Autodesk Inventor part; units mm, degrees
ref_plane "YZ Plane" through (0, 0, 0) normal (1, 0, 0) x (0, 1, 0)
ref_plane "XZ Plane" through (0, 0, 0) normal (0, 1, 0) x (-1, 0, 0)
ref_plane "XY Plane" through (0, 0, 0) normal (0, 0, 1) x (1, 0, 0)
sketch "Sketch1" plane through (0, 0, 0) normal (0, 0, 1) x (1, 0, 0)
  line L0 (0, 0) -> (25, 0)
  line L1 (25, 0) -> (25, 3)
  line L2 (0, 3) -> (25, 3)
  line L3 (0, 0) -> (0, 3)
  line L4 (0.2071, -72) -> (11, -72)
  line L5 (0.2071, -69) -> (11, -69)
  line L6 (25, -69) -> (50, -69)
  line L7 (25, 0) -> (50, 0)
  line L8 (-25, 0) -> (0, 0)
  line L9 (-22, 0) -> (-22, -10.8146)
  line L10 (-25, -22) -> (-25, -47)
  line L11 (-25, -47) -> (-22, -47)
  line L12 (-22, -10.8146) -> (-22, -58.1854)
  line L13 (-25, -22) -> (-22, -22)
  line L14 (-22, -58.1854) -> (-22, -69)
  line L15 (-25, -69) -> (0, -69)
  line L16 (50, 0) -> (50, -22)
  line L17 (50, -22) -> (47, -22)
  line L18 (47, -22) -> (47, -47)
  line L19 (47, -47) -> (50, -47)
  line L20 (50, -47) -> (50, -69)
  line L21 (50, 0) -> (25, 0)
  line L22 (25, 3) -> (25, 0)
  line L23 (25, 3) -> (0, 3)
  line L24 (0, 3) -> (0, 0)
  line L25 (-22, -10.8146) -> (-22, 0)
  line L26 (-22, 0) -> (0, 0)
  line L27 (-22, -22) -> (-25, -22)
  line L28 (-25, -22) -> (-25, -47)
  line L29 (-22, -47) -> (-25, -47)
  line L30 (-22, -58.1854) -> (-22, -69)
  line L31 (-22, -69) -> (0, -69)
  line L32 (0, -72) -> (0, -69)
  line L33 (0, -72) -> (25, -72)
  line L34 (25, -72) -> (25, -69)
  line L35 (25, -69) -> (50, -69)
  line L36 (11, -72) -> (11, -69)
  line L37 (0.2071, -69) -> (0.2071, -72)
  dimension "d0" = 3
extrude "Extrusion1" add sketch "Sketch1" along normal blind 3
sketch "Sketch2" plane through (0, 0, 3) normal (0, 0, 1) x (1, 0, 0)
  line L0 (-25, -22) -> (-25, -47)
  line L1 (-25, -34.5) -> (7, -34.5)
  line L2 (-25, -34.5) -> (-14, -34.5)
  circle A0 centre (-14, -34.5) radius 21
  circle A1 centre (-14, -34.5) radius 25
  point P0 (0, 0)
  dimension "d3" = 32
  dimension "d4" = 11
  dimension "d5" = 4
extrude "Extrusion2" cut sketch "Sketch2" against normal blind 20 contours A0 | A1
sketch "Sketch3" plane through (0, 0, 3) normal (0, 0, 1) x (1, 0, 0)
  line L0 (-1.2929, -65) -> (30.2929, -65)
  line L1 (-4.5, -67) -> (-4.5, -65)
  line L2 (33.5, -67) -> (33.5, -65)
  line L3 (30.6464, -65) -> (33.5, -65)
  line L4 (30.6464, -65) -> (30.2929, -65)
  line L5 (30.2929, -67) -> (30.6464, -67)
  line L6 (33.5, -67) -> (30.6464, -67)
  line L7 (30.2929, -67) -> (-1.2929, -67)
  arc A0 (-22, -58.1854) -> (-22, -10.8146) centre (-14, -34.5) ccw
  line L8 (-22, -58.1854) -> (-22, -69)
  line L9 (-22, -69) -> (0, -69)
  line L10 (0, -69) -> (0, -72)
  line L11 (50, -69) -> (50, -47)
  line L12 (50, -47) -> (47, -47)
  line L13 (47, -47) -> (47, -22)
  line L14 (47, -22) -> (50, -22)
  line L15 (50, -22) -> (50, 0)
  line L16 (50, 0) -> (25, 0)
  line L17 (25, 0) -> (25, 3)
  line L18 (25, 3) -> (0, 3)
  line L19 (0, 3) -> (0, 0)
  line L20 (0, 0) -> (-22, 0)
  line L21 (-22, 0) -> (-22, -10.8146)
  line L22 (-4.5, -65) -> (-1.6464, -65)
  line L23 (-1.2929, -65) -> (-1.6464, -65)
  line L24 (-1.6464, -67) -> (-4.5, -67)
  line L25 (-1.6464, -67) -> (-1.2929, -67)
  line L26 (0, -72) -> (25, -72)
  line L27 (25, -69) -> (50, -69)
  line L28 (25, -72) -> (25, -69)
extrude "Extrusion3" cut sketch "Sketch3" against normal blind 3 contours L0 L4 L3 L2 L6 L5 L7 L25 L24 L1 L22 L23
sketch "Sketch4" plane through (0, 0, 3) normal (0, 0, 1) x (1, 0, 0)
  line L0 (47, -47) -> (47, -22)
  line L1 (47, -34.5) -> (34.3, -34.5)
  line L2 (34.3, -34.5) -> (34.3, -36)
  line L3 (34.3, -36) -> (34.3, -33)
  line L4 (34.3, -33) -> (47, -33)
  line L5 (47, -33) -> (47, -36)
  line L6 (47, -36) -> (34.3, -36)
  line L7 (40.65, -36) -> (40.65, -38)
  line L8 (40.65, -38) -> (38.15, -38)
  line L9 (38.15, -38) -> (38.15, -31)
  line L10 (38.15, -31) -> (40.65, -31)
  line L11 (40.65, -31) -> (40.65, -36)
  line L12 (25, 3) -> (0, 3)
  line L13 (50, 0) -> (25, 0)
  line L14 (0, 0) -> (-22, 0)
  line L15 (25, -69) -> (50, -69)
  line L16 (0, -72) -> (25, -72)
  line L17 (-22, -69) -> (0, -69)
  line L18 (50, 0) -> (25, 0)
  line L19 (37.5, 0) -> (37.5, -12.7)
  line L20 (37.5, -12.7) -> (39, -12.7)
  line L21 (39, -12.7) -> (36, -12.7)
  line L22 (36, -12.7) -> (36, 0)
  line L23 (39, 0) -> (39, -12.7)
  line L24 (36, -6.35) -> (34, -6.35)
  line L25 (34, -6.35) -> (34, -8.85)
  line L26 (34, -8.85) -> (41, -8.85)
  line L27 (41, -8.85) -> (41, -6.35)
  line L28 (41, -6.35) -> (36, -6.35)
  line L29 (50, -69) -> (25, -69)
  line L30 (37.5, -69) -> (37.5, -56.3)
  line L31 (37.5, -56.3) -> (39, -56.3)
  line L32 (39, -56.3) -> (36, -56.3)
  line L33 (36, -56.3) -> (36, -69)
  line L34 (39, -69) -> (39, -56.3)
  line L35 (36, -62.65) -> (34, -62.65)
  line L36 (34, -62.65) -> (34, -60.15)
  line L37 (34, -60.15) -> (41, -60.15)
  line L38 (41, -60.15) -> (41, -62.65)
  line L39 (41, -62.65) -> (36, -62.65)
  line L40 (-4.5, -65) -> (33.5, -65)
  line L41 (33.5, -65) -> (33.5, -67)
  line L42 (33.5, -67) -> (-4.5, -67)
  line L43 (-4.5, -67) -> (-4.5, -65)
  arc A0 (-22, -58.1854) -> (-22, -10.8146) centre (-14, -34.5) ccw
  line L44 (-22, -58.1854) -> (-22, -69)
  line L45 (-22, -69) -> (0, -69)
  line L46 (0, -69) -> (0, -72)
  line L47 (0, -72) -> (25, -72)
  line L48 (25, -69) -> (50, -69)
  line L49 (50, -69) -> (50, -47)
  line L50 (50, -47) -> (47, -47)
  line L51 (47, -47) -> (47, -22)
  line L52 (47, -22) -> (50, -22)
  line L53 (50, -22) -> (50, 0)
  line L54 (50, 0) -> (25, 0)
  line L55 (25, 0) -> (25, 3)
  line L56 (25, 3) -> (0, 3)
  line L57 (0, 3) -> (0, 0)
  line L58 (0, 0) -> (-22, 0)
  line L59 (-22, 0) -> (-22, -10.8146)
  circle A1 centre (12.5, 1.5) radius 1.5
  line L60 (39, -56.3) -> (36, -56.3)
  line L61 (36, -56.3) -> (36, -69)
  line L62 (36, -69) -> (39, -69)
  line L63 (39, -69) -> (39, -56.3)
  circle A2 centre (12.5, -70.5) radius 1.5
  line L64 (25, -72) -> (25, -69)
  arc A3 (42.9741, -36.0257) -> (30.0259, -20.7829) centre (36.5, -28.4043) ccw
  line L65 (26.9692, -49.6214) -> (42.9741, -36.0257)
  arc A4 (14.0209, -34.3786) -> (26.9692, -49.6214) centre (20.4951, -42) ccw
  line L66 (30.0259, -20.7829) -> (14.0209, -34.3786)
  dimension "d10" = 12.7
  dimension "d11" = 1.5
  dimension "d12" = 3
  dimension "d13" = 2
  dimension "d14" = 2.5
  dimension "d15" = 7
  dimension "d16" = 12.7
  dimension "d17" = 1.5
  dimension "d18" = 3
  dimension "d19" = 2
  dimension "d20" = 2.5
  dimension "d21" = 7
  dimension "d22" = 3
  dimension "d25" = 3
extrude "Extrusion4" cut sketch "Sketch4" against normal blind 25.4 contours A1 | A2 | L15 L30 L39 L34 | L15 L33 L39 L30 | L39 L30 L37 L34 | L34 L37 L38 L39 | L39 L33 L37 L30 | L37 L30 L31 L34 | L35 L36 L37 L33 | L37 L33 L32 L30 | L23 L28 L19 L13 | L19 L28 L22 L13 | L28 L27 L26 L23 | L23 L26 L19 L28 | L19 L26 L22 L28 | L23 L20 L19 L26 | L22 L26 L25 L24 | L19 L21 L22 L26
properties part number "pared frontal 2"
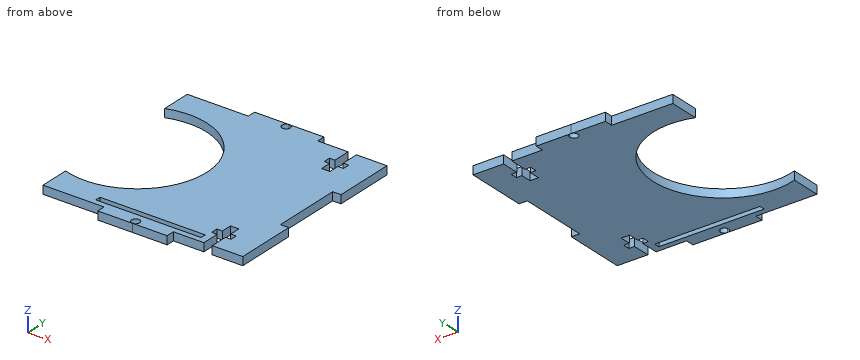
Geometry: final body of the model. Coordinates: model frame, mm. Give positions to 0.01 mm unless a question says otherwise; leave off trailing zeros. Order: outer loops, then holes, each group sorted by start corner. A loop starts at its lowest first (then second) coordinate and runs counter-clockwise, first axis right, second up. Notation, with made-up numbers: (-37, -22.5) -> (14, -22.5) arc R29 ccw to (14, 0.5) -> close; hole circle Ø8 at (80, -10.75). An arc over 180 degrees is marked (long way). Write each question's results on one line, items separated by ' | '. Start each with the question number.
1) Line query: line 1 (X direction, y = -70.5, z = 1.9); line 2 (Y direction, x = -10, z = 1.3); line 3 (X direction, y = -34.5, z = 0.8). Output: solid intervals per line, ascending. Write a range as from..to.
2) Section B-B (y = -4.5). Return loops of the section in (x, z).
3) Section A-A (x = -7). Return loops of the section in (y, z).
4) First-contact query: pin 1 (0.6 mm diameter, centred on x = 35, z = 1, fed in from +Y); pin 2 (1 mm diameter, centred on x = 38, y = -57, fed in from -Z). Flat tips, straight axial feed; report the tip coordinate or a pass-through.
5) Section D-D (y = -42.5). Return loops of the section in (x, z), then the cut area to 3 significant figures.
Calculated:
1) line 1: 0..11, 14..25 | line 2: -69..-59.18, -9.82..0 | line 3: 11..47
2) outline: (-22, 0) -> (36, 0) -> (36, 3) -> (-22, 3) -> close; (39, 0) -> (50, 0) -> (50, 3) -> (39, 3) -> close
3) outline: (-69, 0) -> (-58.5, 0) -> (-58.5, 3) -> (-69, 3) -> close; (-10.5, 0) -> (0, 0) -> (0, 3) -> (-10.5, 3) -> close
4) pin 1: y = 0 | pin 2: through
5) outline: (9.69, 0) -> (47, 0) -> (47, 3) -> (9.69, 3) -> close | area: 112 mm2
